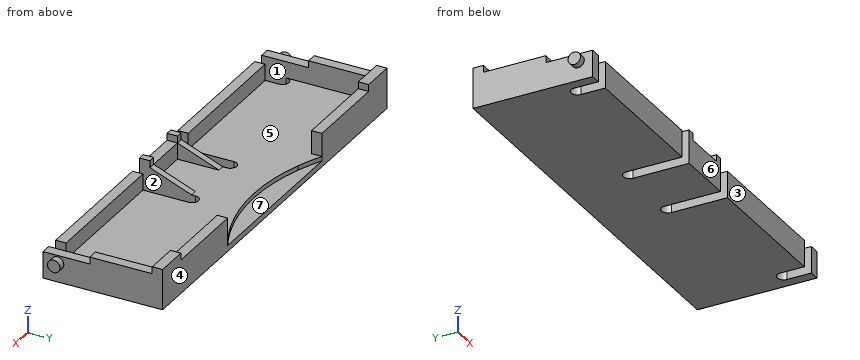
```python
from build123d import *

# Parameters (mm, degrees)
F0_W      = 59.5
F0_H      = 17.25
F1_DEPTH  = 4.85
F2_T      = -1.5
F3_W      = 1.85
F3_H      = 1.5
F4_DEPTH  = 4.851
F6_DEPTH  = 4
F8_DEPTH  = 3.351
F9_W      = 1.5
F9_H      = 6.75
F10_DEPTH = 1
F11_W     = 4.85
F11_H     = 1.5
F12_DEPTH = 1
F13_W     = 1.5
F13_H     = 1
F14_DEPTH = 1
F15_W     = 1.5
F15_H     = 1
F16_DEPTH = 1
F17_R     = 0.9
F18_DEPTH = 1
F19_R     = 0.9
F20_DEPTH = 1


with BuildPart() as f1:
    # F0 (on Top) → F1 (new body)
    with BuildSketch(Plane.XY):
        with Locations((-29.75, 8.625)):
            Rectangle(F0_W, F0_H)
    extrude(amount=F1_DEPTH)

    # F2
    f2_openings = [f1.faces().sort_by_distance(p)[0] for p in [
        (-29.75, 8.625, 4.85),
    ]]
    offset(amount=F2_T, openings=f2_openings)

    # F3 (on face) → F4 (cut, through all)
    with BuildSketch(Plane.XY.offset(4.85)):
        with BuildLine():
            Line((-35.75, 8.075), (-35.75, 1.5))
            Line((-35.75, 1.5), (-33.9, 1.5))
            Line((-33.9, 1.5), (-33.9, 8.075))
            ThreePointArc((-33.9, 8.075), (-34.825, 9), (-35.75, 8.075))
        make_face()
        with Locations((-34.825, 0.75)):
            Rectangle(F3_W, F3_H)
        with BuildLine():
            Line((-58, 1.5), (-56.15, 1.5))
            Line((-56.15, 1.5), (-56.15, 3.5))
            ThreePointArc((-56.15, 3.5), (-57.075, 4.425), (-58, 3.5))
            Line((-58, 3.5), (-58, 1.5))
        make_face()
        with Locations((-57.075, 0.75)):
            Rectangle(F3_W, F3_H)
        with BuildLine():
            Line((-25.6, 8.075), (-25.6, 1.5))
            Line((-25.6, 1.5), (-23.75, 1.5))
            Line((-23.75, 1.5), (-23.75, 8.075))
            ThreePointArc((-23.75, 8.075), (-24.675, 9), (-25.6, 8.075))
        make_face()
        with Locations((-24.675, 0.75)):
            Rectangle(F3_W, F3_H)
        with BuildLine():
            Line((-1.5, 1.5), (-1.5, 3.5))
            ThreePointArc((-1.5, 3.5), (-2.425, 4.425), (-3.35, 3.5))
            Line((-3.35, 3.5), (-3.35, 1.5))
            Line((-3.35, 1.5), (-1.5, 1.5))
        make_face()
        with Locations((-2.425, 0.75)):
            Rectangle(F3_W, F3_H)
    extrude(amount=-F4_DEPTH, mode=Mode.SUBTRACT)

    # F5 (on face) → F6 (cut)
    with BuildSketch(Plane.XY.offset(4.85)):
        with BuildLine():
            Line((-20.7847894615, 15.75), (-38.7152105385, 15.75))
            ThreePointArc((-38.7152105385, 15.75), (-29.75, 14.25), (-20.7847894615, 15.75))
        make_face()
        with BuildLine():
            Line((-17.25, 17.25), (-42.25, 17.25))
            ThreePointArc((-42.25, 17.25), (-40.508778549, 16.4383219778), (-38.7152105385, 15.75))
            Line((-38.7152105385, 15.75), (-20.7847894615, 15.75))
            ThreePointArc((-20.7847894615, 15.75), (-18.991221451, 16.4383219778), (-17.25, 17.25))
        make_face()
    extrude(amount=-F6_DEPTH, mode=Mode.SUBTRACT)

    # F7 (on face) → F8 (cut, through all)
    with BuildSketch(Plane.XY.offset(1.5)):
        with BuildLine():
            Line((-42.25, 17.25), (-42.25, 15.75))
            Line((-42.25, 15.75), (-38.7152105385, 15.75))
            ThreePointArc((-38.7152105385, 15.75), (-40.508778549, 16.4383219778), (-42.25, 17.25))
        make_face()
        with BuildLine():
            ThreePointArc((-17.25, 17.25), (-18.991221451, 16.4383219778), (-20.7847894615, 15.75))
            Line((-20.7847894615, 15.75), (-17.25, 15.75))
            Line((-17.25, 15.75), (-17.25, 17.25))
        make_face()
    extrude(amount=F8_DEPTH, mode=Mode.SUBTRACT)

    # F9 (on face) → F10 (cut)
    with BuildSketch(Plane.XY.offset(4.85)):
        with Locations((-58.75, 3.375)):
            Rectangle(F9_W, F9_H)
        Polygon((-59.5, 6.75), (-60.5477912843, 6.75), (-60.5477912843, -8.7434453119), (1.7196297206, -8.7434453119), (1.7196297206, 6.75), (-58, 6.75), (-58, 0), (-59.5, 0), align=None)
    extrude(amount=-F10_DEPTH, mode=Mode.SUBTRACT)

    # F11 (on face) → F12 (join)
    with BuildSketch(Plane.XY.offset(4.85)):
        Polygon((-54.65, 17.25), (-59.5, 17.25), (-59.5, 15.75), (-58, 15.75), (-54.65, 15.75), align=None)
        with Locations((-2.425, 16.5)):
            Rectangle(F11_W, F11_H)
    extrude(amount=F12_DEPTH)

    # F13 (on face) → F14 (join)
    with BuildSketch(Plane(origin=(-33.9, 0, 0), x_dir=(0, -1, 0), z_dir=(-1, 0, 0))):
        Polygon((-1.5, 1.5), (-1.5, 3.85), (-7.5, 1.5), align=None)
        with Locations((-0.75, 4.35)):
            Rectangle(F13_W, F13_H)
    extrude(amount=-F14_DEPTH)

    # F15 (on face) → F16 (join)
    with BuildSketch(Plane.YZ.offset(-25.6)):
        with Locations((0.75, 4.35)):
            Rectangle(F15_W, F15_H)
        Polygon((7.5, 1.5), (1.5, 3.85), (1.5, 1.5), align=None)
    extrude(amount=-F16_DEPTH)

    # F17 (on face) → F18 (join)
    with BuildSketch(Plane.YZ):
        with Locations((2.1, 2.75)):
            Circle(F17_R)
    extrude(amount=F18_DEPTH)

    # F19 (on face) → F20 (join)
    with BuildSketch(Plane(origin=(-59.5, 0, 0), x_dir=(0, -1, 0), z_dir=(-1, 0, 0))):
        with Locations((-2.1, 2.75)):
            Circle(F19_R)
    extrude(amount=F20_DEPTH)


solid = f1.part
```
Model file for the job. Use its own axes, mm. Face numbers are marked on the shaded views. A direction names the side the tool comes from. Coordinates: 2 decimals unless noted, no trailing zeros. Order: outer loops, then holes, each group sorted by start corner. A loop starts at its lowest first (then second) coordinate and runs counter-clockwise, first axis right, second up. Notation, with made-up numbers: (67, -10) - (104, -10) arc R20 ccw to (104, 6) - close; hole circle Ø9 at (58, 50.25). An arc over 180 degrees is marked (long way). Return JSON: item names as keys, results as strings. Group by question number.
1) Flat gauge pins, fed straight in: P1, Ø0.8, axis at y = 16, z = 5.5, coming from the -X side; P2, Ø1.2, axis at x = -1, y = 10.5, coming from the +Z side; P3, Ø0.8, axis at x = -29, y = 0.5, coming from the +Z side; P4, Ø6, axis at x = -6, y = 8, coming from the -Z side. Where does each tip first touch, or does it go through?
2) Tool access for the marked faces 1, 2 and 3: list every direction of +Z, -Z, +X, -X, +Y, -Y with a clear straight run to the whole face (end or side of a thin tool).
3) Saw through at C-C, the plane y = 2.1. Count the separate pieces of the cut face and the enclosed holes in it, plus the area to 3 significant figures.
4) Saw through at A-A, the plane x = -45. Write the cut outline in (y, z).
5) Mould opens along Y. For the marked faces 4, 5, 6 and 7 say: released by +Y, released by -Y, zero draft, split by the parting line, or undercut.
6) Probe line 1 (X direction, y = 1.5, z = 1.2); line 2 (X direction, y = 5.5, z = 3.4); line 3 (Y direction, x = -43.5, z = 2.6). List the from-to ranges inside material, lowest first. Write a range as from..to.
7) Saw through at B-B, the plane y = 10.5. Write the cut outline in (x, z).
Values found:
{
 "1": {"P1": "stops at x = -59.5", "P2": "stops at z = 4.85", "P3": "stops at z = 3.85", "P4": "stops at z = 0"},
 "2": {"face 1": "+Z, -Y", "face 2": "+Z, -Z, -Y", "face 3": "+Z, -Z, +X, -X, -Y"},
 "3": {"separate pieces": "5", "enclosed holes": "0", "area": "93.0 mm²"},
 "4": {"outline": "(0, 0) - (17.25, 0) - (17.25, 4.85) - (15.75, 4.85) - (15.75, 1.5) - (1.5, 1.5) - (1.5, 3.85) - (0, 3.85) - close"},
 "5": {"face 4": "released by +Y", "face 5": "undercut", "face 6": "released by -Y", "face 7": "zero draft"},
 "6": {"line 1": "x = -59.5..-58, -56.15..-35.75, -33.9..-25.6, -23.75..-3.35, -1.5..0", "line 2": "x = -59.5..-58, -1.5..0", "line 3": "y = 0..1.5, 15.75..17.25"},
 "7": {"outline": "(-59.5, 0) - (0, 0) - (0, 4.85) - (-1.5, 4.85) - (-1.5, 1.5) - (-58, 1.5) - (-58, 4.85) - (-59.5, 4.85) - close"}
}
